```python
from build123d import *

# Parameters (mm, degrees)
SKETCH1_W           = 38.1
SKETCH1_H           = 95.25
BOSS_EXTRUDE1_DEPTH = 6.35
SKETCH2_W           = 20.32
SKETCH2_H           = 40.64
CUT_EXTRUDE1_DEPTH  = 6.35


with BuildPart() as part:
    # Sketch1 → Boss-Extrude1 (new body)
    with BuildSketch(Plane.XY):
        with Locations((19.05, 47.625)):
            Rectangle(SKETCH1_W, SKETCH1_H)
    extrude(amount=BOSS_EXTRUDE1_DEPTH)

    # Sketch2 → Cut-Extrude1 (cut)
    with BuildSketch(Plane(origin=(0, 0, 0), x_dir=(-1, 0, 0), z_dir=(0, 0, -1))):
        with Locations((-18.415, 59.725)):
            Rectangle(SKETCH2_W, SKETCH2_H)
        with BuildLine():
            Line((-25.165, 83.725), (-25.165, 85.725))
            ThreePointArc((-25.165, 85.725), (-23.415, 87.475), (-21.665, 85.725))
            Line((-21.665, 85.725), (-21.665, 83.725))
            ThreePointArc((-21.665, 83.725), (-23.415, 81.975), (-25.165, 83.725))
        make_face()
        with BuildLine():
            Line((-15.165, 83.725), (-15.165, 85.725))
            ThreePointArc((-15.165, 85.725), (-13.415, 87.475), (-11.665, 85.725))
            Line((-11.665, 85.725), (-11.665, 83.725))
            ThreePointArc((-11.665, 83.725), (-13.415, 81.975), (-15.165, 83.725))
        make_face()
        with BuildLine():
            Line((-21.665, 35.725), (-21.665, 33.725))
            ThreePointArc((-21.665, 33.725), (-23.415, 31.975), (-25.165, 33.725))
            Line((-25.165, 33.725), (-25.165, 35.725))
            ThreePointArc((-25.165, 35.725), (-23.415, 37.475), (-21.665, 35.725))
        make_face()
        with BuildLine():
            Line((-11.665, 35.725), (-11.665, 33.725))
            ThreePointArc((-11.665, 33.725), (-13.415, 31.975), (-15.165, 33.725))
            Line((-15.165, 33.725), (-15.165, 35.725))
            ThreePointArc((-15.165, 35.725), (-13.415, 37.475), (-11.665, 35.725))
        make_face()
    extrude(amount=-CUT_EXTRUDE1_DEPTH, mode=Mode.SUBTRACT)


solid = part.part
```
Could you check a few things on this model? Use its own coordinates, in mm. A direction names the side the tool comes from. Coordinates: 2 decimals unless noted, no trailing zeros. Write each loop counter-clockwise with the first axis right and the second up, starting at its lowest first coordinate (ties: lowest second). Pieces come first, ordered by that corner, then holes. Notation, with made-up numbers: (32, 21) -> (56, 21) arc R12 cw to (56, 34) -> close; hole circle Ø1 at (25, -18.75). An arc over 180 degrees is marked (long way). One line per question, with ' | ' between items. Start each with the question number.
1. Please list where these lines run through material, in increasing order: line 1 along Y through (x, z) = (18.5, 2.25) (3 decimals); line 2 along X through (y, z) = (53.5, 3) (3 decimals); line 3 along Y through (x, z) = (25, 4.5) (3 decimals).
2. If we section it at C-C (z = 2.75): Please give me the cut outline in (x, y) (3 decimals), and give its area (3 significant figures).
3. Will these pins go through, and if not, where does the flat tip stop? P1, Ø10, axis at x = 29.5, y = 56.5, coming from the -Z side; P2, Ø8, axis at x = 15, y = 60.5, coming from the +Z side.
4. If we section it at B-B (y = 67): Please give me the cut outline in (x, z) (3 decimals).
5. If we section it at A-A (x = 17): Please give me the cut outline in (y, z) (3 decimals).
6. For faces 1 (the face through (21.665, 85, 3)), 2 (the face through (19, 38, 6.35)), which set-ups out of +Z, -Z, +X, -X, +Y, -Y let a thin tool reach every point of the face, with its end or its side?
7. Thinking about a two-plate mould opening in X: for faces 3 (the face through (19, 95.25, 3)), 4 (the face through (0, 47, 3)), 5 (the face through (13.453, 87.475, 3.131)), which applies, pulls with the +X half, pulls with the -X half, needs draft (parallel to the pull), parting line crosses it, or undercut?
Return value:
1) line 1: y = 0 to 39.405, 80.045 to 95.25 | line 2: x = 0 to 8.255, 28.575 to 38.1 | line 3: y = 0 to 32.983, 36.467 to 39.405, 80.045 to 82.983, 86.467 to 95.25
2) outline: (0, 0) -> (38.1, 0) -> (38.1, 95.25) -> (0, 95.25) -> close; hole (8.255, 39.405) -> (28.575, 39.405) -> (28.575, 80.045) -> (8.255, 80.045) -> close; hole (11.665, 33.725) arc R1.75 ccw to (15.165, 33.725) -> (15.165, 35.725) arc R1.75 ccw to (11.665, 35.725) -> close; hole (11.665, 83.725) arc R1.75 ccw to (15.165, 83.725) -> (15.165, 85.725) arc R1.75 ccw to (11.665, 85.725) -> close; hole (21.665, 33.725) arc R1.75 ccw to (25.165, 33.725) -> (25.165, 35.725) arc R1.75 ccw to (21.665, 35.725) -> close; hole (21.665, 83.725) arc R1.75 ccw to (25.165, 83.725) -> (25.165, 85.725) arc R1.75 ccw to (21.665, 85.725) -> close | area: 2,740 mm²
3) P1: stops at z = 0 | P2: passes through
4) outline: (0, 0) -> (8.255, 0) -> (8.255, 6.35) -> (0, 6.35) -> close; (28.575, 0) -> (38.1, 0) -> (38.1, 6.35) -> (28.575, 6.35) -> close
5) outline: (0, 0) -> (39.405, 0) -> (39.405, 6.35) -> (0, 6.35) -> close; (80.045, 0) -> (95.25, 0) -> (95.25, 6.35) -> (80.045, 6.35) -> close
6) face 1: +Z, -Z | face 2: +Z, +X, -X, +Y, -Y
7) face 3: needs draft | face 4: pulls with the -X half | face 5: undercut
